Work out the finished part from the listing and answer in its coordinate system (mm). A direction names the side the tool comes from. Coordinates: 2 decimals unless noted, no trailing zeros. Loops run counter-clockwise (first coordinate to the right, second up) from the corner with the lowest first, then second, coordinate; pieces in that order, holes last.
```python
from build123d import *

# Parameters (mm, degrees)
F2_R     = 139.7
F2_R_2   = 2.9765625
F3_DEPTH = 19.05
F4_SIZE  = 1.5875
F6_W     = 12.7
F6_H     = 5.55625
F7_DEPTH = 38.1
F8_W     = 114.3
F8_H     = 63.5
F8_R     = 2.9765625
F9_DEPTH = 19.051


# Not quite as in the source:
# - a variable given as a bare number and used for a length is read in inches; the dataset says mm whatever the document's units were


with BuildPart() as f3:
    # F2 (on Top) → F3 (new body)
    with BuildSketch(Plane.XY):
        Circle(F2_R)
        Circle(F2_R_2, mode=Mode.SUBTRACT)
    extrude(amount=F3_DEPTH)

    # F4
    f4_edges = [f3.edges().sort_by_distance(p)[0] for p in [
        (-139.7, 0, 19.05),
        (-139.7, 0, 0),
    ]]
    chamfer(f4_edges, length=F4_SIZE)

    # F6 (on offset) → F7 (cut)
    with BuildSketch(Plane.XZ.offset(139.7)):
        with Locations((0, 16.271875)):
            Rectangle(F6_W, F6_H)
    extrude(amount=-F7_DEPTH, mode=Mode.SUBTRACT)

    # F8 (on face) → F9 (cut, through all)
    with BuildSketch(Plane.XY.offset(19.05)):
        Rectangle(F8_W, F8_H)
        Circle(F8_R, mode=Mode.SUBTRACT)
    extrude(amount=-F9_DEPTH, mode=Mode.SUBTRACT)


solid = f3.part
```
1. Straight lines are drawn through the part: probe 1 along X at (y, z) = (19, 5.25); probe 2 along Y at (x, z) = (28, 8.5); probe 3 along Y at (x, z) = (25, 13.25). For each, find the intervals that lie inside material, in ascending order.
2. A cutting plane is placed at A-A, the plane x = 0. Give the vertices of the cut face in (y, z).
3. Each of these flat-tipped pins is pushed along its axis until it touches: P1, Ø5, axis at x = -52, z = 12, coming from the -Y side; P2, Ø4.5, axis at x = -2.5, z = 16.5, coming from the -Y side; P3, Ø4, axis at y = 85.5, z = 11, coming from the +X side; P4, Ø5, axis at x = -74, y = 107.5, coming from the -Z side. Where does it stop, or does it pass through?
4. Determine the mould class of faces 3 (the flat face through (0, -121, 13.494)), 4 (the cylindrical face through (-110.86, -85.01, 9.41)), 5 (the flat face through (-2, 33, 0)) for opening direction X: released by +X, released by -X, zero draft, split by the parting line, or undercut.
5. A cutting plane is placed at B-B, the plane z = 5.5. Give the vertices of the cut face in (x, y), then the cut area to 3 significant figures.
6. For faces 1 (the flat face through (-2, 33, 19.05)), 2 (the flat face through (-1, -31.75, 10)), determine the directions among +Z, -Z, +X, -X, +Y, -Y from which every point of the face is accessible in a straight line to the end or side of a thin tool.
Answers below:
1. probe 1: x = -138.4 to -57.15, 57.15 to 138.4
1. probe 2: y = -136.87 to -31.75, 31.75 to 136.87
1. probe 3: y = -137.44 to -31.75, 31.75 to 137.44
2. outline: (-139.7, 1.59) - (-138.11, 0) - (-31.75, 0) - (-31.75, 19.05) - (-101.6, 19.05) - (-101.6, 13.49) - (-139.7, 13.49) - close; (31.75, 0) - (138.11, 0) - (139.7, 1.59) - (139.7, 17.46) - (138.11, 19.05) - (31.75, 19.05) - close
3. P1: stops at y = -130.64
3. P2: stops at y = -101.6
3. P3: stops at x = 112
3. P4: stops at z = 0
4. face 3: undercut
4. face 4: split by the parting line
4. face 5: zero draft
5. outline: circle Ø279.4 at (0, 0); hole (-57.15, -31.75) - (57.15, -31.75) - (57.15, 31.75) - (-57.15, 31.75) - close
5. area: 54,100 mm2
6. face 1: +Z, +X, -X, +Y, -Y
6. face 2: +Z, -Z
